Work out the finished part from the listing and answer in its coordinate system (mm). A direction names the side the tool comes from. Coordinates: 2 decimals unless noted, no trailing zeros. Loops run counter-clockwise (first coordinate to the right, second up) from the corner with the lowest first, then second, coordinate; pieces in that order, holes last. Notation, with made-up numbers: (32, -19.5) -> (40, -19.5) arc R34 ccw to (40, 13.5) -> close; hole circle Ø11 at (87, 32). An arc over 180 degrees is marked (long way). Use a Markdown table: item, result. Add a question column.
```python
from build123d import *

# Parameters (mm, degrees)
SKICA1_W                = 35
SKICA1_H                = 15
SKICA1_W_2              = 40
SKICA1_H_2              = 4
SKICA1_R                = 1.625
SKICA1_W_3              = 7
SKICA1_H_3              = 11
SKICA1_W_4              = 4
SKICA1_H_4              = 20
P_IDAT_VYSUNUT_M1_DEPTH = 4


with BuildPart() as part:
    # Skica1 → Přidat vysunutím1 (new body)
    with BuildSketch(Plane(origin=(0, 0, 0), x_dir=(1, 0, 0), z_dir=(0, 1, 0))):
        with BuildLine():
            Line((-114, 97.488460856), (-114, 20))
            Line((-114, 20), (-90, 20))
            Line((-90, 20), (-90, 24))
            Line((-90, 24), (-70, 24))
            Line((-70, 24), (-70, 20))
            Line((-70, 20), (-50, 20))
            Line((-50, 20), (-50, 24))
            Line((-50, 24), (-30, 24))
            Line((-30, 24), (-30, 20))
            Line((-30, 20), (-24, 20))
            Line((-24, 20), (-24, -20))
            Line((-24, -20), (-30, -20))
            Line((-30, -20), (-30, -24))
            Line((-30, -24), (-50, -24))
            Line((-50, -24), (-50, -20))
            Line((-50, -20), (-70, -20))
            Line((-70, -20), (-70, -24))
            Line((-70, -24), (-90, -24))
            Line((-90, -24), (-90, -20))
            Line((-90, -20), (-114, -20))
            Line((-114, -20), (-114, -97.488460856))
            ThreePointArc((-114, -97.488460856), (0, -150), (114, -97.488460856))
            Line((114, -97.488460856), (114, -20))
            Line((114, -20), (90, -20))
            Line((90, -20), (90, -24))
            Line((90, -24), (70, -24))
            Line((70, -24), (70, -20))
            Line((70, -20), (50, -20))
            Line((50, -20), (50, -24))
            Line((50, -24), (30, -24))
            Line((30, -24), (30, -20))
            Line((30, -20), (24, -20))
            Line((24, -20), (24, 20))
            Line((24, 20), (30, 20))
            Line((30, 20), (30, 24))
            Line((30, 24), (50, 24))
            Line((50, 24), (50, 20))
            Line((50, 20), (70, 20))
            Line((70, 20), (70, 24))
            Line((70, 24), (90, 24))
            Line((90, 24), (90, 20))
            Line((90, 20), (114, 20))
            Line((114, 20), (114, 97.488460856))
            ThreePointArc((114, 97.488460856), (0, 150), (-114, 97.488460856))
        make_face()
        with Locations((0, -132.5)):
            Rectangle(SKICA1_W, SKICA1_H, mode=Mode.SUBTRACT)
        with Locations((0, -71)):
            Rectangle(SKICA1_W_2, SKICA1_H_2, mode=Mode.SUBTRACT)
        with Locations((0, 100.5)):
            Circle(SKICA1_R, mode=Mode.SUBTRACT)
        with Locations((0, 114)):
            Rectangle(SKICA1_W_3, SKICA1_H_3, mode=Mode.SUBTRACT)
        with Locations((0, 132.5)):
            Rectangle(SKICA1_W, SKICA1_H, mode=Mode.SUBTRACT)
        with Locations((-102, 40)):
            Rectangle(SKICA1_W_4, SKICA1_H_4, mode=Mode.SUBTRACT)
        with Locations((-71.064231509, 71.064231509)):
            Circle(SKICA1_R, mode=Mode.SUBTRACT)
        with Locations((-102, 80)):
            Rectangle(SKICA1_W_4, SKICA1_H_4, mode=Mode.SUBTRACT)
        Polygon((-86.974134086, 82.024386618), (-82.024386618, 86.974134086), (-74.246212025, 79.195959493), (-79.195959493, 74.246212025), align=None, mode=Mode.SUBTRACT)
        Polygon((-48.964248531, 109.064212122), (-42.497091804, 111.742996148), (-38.287574048, 101.580321291), (-44.754730775, 98.901537264), align=None, mode=Mode.SUBTRACT)
        with Locations((-38.459684953, 92.849893017)):
            Circle(SKICA1_R, mode=Mode.SUBTRACT)
        with Locations((-102, -40)):
            Rectangle(SKICA1_W_4, SKICA1_H_4, mode=Mode.SUBTRACT)
        with Locations((-102, -80)):
            Rectangle(SKICA1_W_4, SKICA1_H_4, mode=Mode.SUBTRACT)
        with Locations((102, 80)):
            Rectangle(SKICA1_W_4, SKICA1_H_4, mode=Mode.SUBTRACT)
        with Locations((71.064231509, 71.064231509)):
            Circle(SKICA1_R, mode=Mode.SUBTRACT)
        with Locations((102, 40)):
            Rectangle(SKICA1_W_4, SKICA1_H_4, mode=Mode.SUBTRACT)
        with Locations((38.459684953, 92.849893017)):
            Circle(SKICA1_R, mode=Mode.SUBTRACT)
        Polygon((82.024386618, 86.974134086), (86.974134086, 82.024386618), (79.195959493, 74.246212025), (74.246212025, 79.195959493), align=None, mode=Mode.SUBTRACT)
        Polygon((42.497091804, 111.742996148), (48.964248531, 109.064212122), (44.754730775, 98.901537264), (38.287574048, 101.580321291), align=None, mode=Mode.SUBTRACT)
        with Locations((102, -40)):
            Rectangle(SKICA1_W_4, SKICA1_H_4, mode=Mode.SUBTRACT)
        with Locations((102, -80)):
            Rectangle(SKICA1_W_4, SKICA1_H_4, mode=Mode.SUBTRACT)
    extrude(amount=P_IDAT_VYSUNUT_M1_DEPTH)


solid = part.part
```
Item 1: Section A-A (z = 130) is taken. Determine the outline of the cut face in (x, y).
Item 2: Given pin 1 (2 mm diameter, centred on x = -44, y = 2, fed in from -Z); pin 2 (2 mm diameter, centred on x = -102, y = 2, fed in from -Z), each flat-ended and moving along its own axis, determine where each tip first touches the part or whether it passes through.
Item 3: Section C-C (y = 1.95) is taken. Count the separate pieces of the cut face and the enclosed holes in it, then the cut area to 3 significant figures.
Item 4: For a pull along X with two mould halves and no side action, classify faces 1 (the face through (-2, 0, -2)), 2 (the face through (-1.81, 1.97, 149.99)), 3 (the face through (-83.03, 1.97, -78.08)) as +X half, -X half, draft (parallel to the pull), parting line (faces both ways), or undercut.
Item 5: Section B-B (x = -65) is taken. Determine the outline of the cut face in (y, z).
Item 6: For faces 4 (the face through (83.14, 1.97, -78.19)), 5 (the face through (1.81, 1.97, -149.99)), determine the directions among +Z, -Z, +X, -X, +Y, -Y from which every point of the face is accessible in a straight line to the end or side of a thin tool.
Item 7: Find the intervals of material crossed by probe 1 along X at (y, z) = (0.95, -23); probe 2 along X at (y, z) = (0.9, -89); probe 3 along Z at (x, y) = (-10, 2.75), in increasing order.
Output:
| question | item | result |
|---|---|---|
| 1 | outline | (-74.83, 0) -> (-17.5, 0) -> (-17.5, 4) -> (-74.83, 4) -> close; (17.5, 0) -> (74.83, 0) -> (74.83, 4) -> (17.5, 4) -> close |
| 2 | pin 1 | stops at z = -143.7 |
| 2 | pin 2 | stops at z = -110.9 |
| 3 | separate pieces | 1 |
| 3 | enclosed holes | 21 |
| 3 | area | 51,000 mm2 |
| 4 | face 1 | draft |
| 4 | face 2 | parting line |
| 4 | face 3 | undercut |
| 5 | outline | (0, -135.19) -> (4, -135.19) -> (4, -20) -> (0, -20) -> close; (0, 20) -> (4, 20) -> (4, 135.19) -> (0, 135.19) -> close |
| 6 | face 4 | +Y, -Y |
| 6 | face 5 | -Z, +Y, -Y |
| 7 | probe 1 | x = -114 to -90, -70 to -50, -30 to 30, 50 to 70, 90 to 114 |
| 7 | probe 2 | x = -114 to -104, -100 to 100, 104 to 114 |
| 7 | probe 3 | z = -149.67 to -140, -125 to 69, 73 to 125, 140 to 149.67 |
